```python
from build123d import *

# Parameters (mm, degrees)
SKETCH1_W           = 21.5
SKETCH1_H           = 43
BOSS_EXTRUDE1_DEPTH = 5
CUT_EXTRUDE1_DEPTH  = 5
SKETCH7_W           = 18.5
SKETCH7_H           = 15
BOSS_EXTRUDE2_DEPTH = 5
SKETCH8_R           = 1.175
CUT_EXTRUDE4_DEPTH  = 8
CUT_EXTRUDE5_REACH  = 38.644
SKETCH11_R          = 1.25
CUT_EXTRUDE6_REACH  = 38.644
SKETCH3_R           = 1.5
SKETCH12_R          = 2.25
CUT_EXTRUDE7_DEPTH  = 2
CHAMFER1_SIZE       = 8
CUT_EXTRUDE8_REACH  = 38.644
FILLET4_R           = 2
FILLET5_R           = 5
SKETCH17_W          = 10
SKETCH17_H          = 4
BOSS_EXTRUDE3_DEPTH = 11
FILLET6_R           = 2


with BuildPart() as part:
    # Sketch1 → Boss-Extrude1 (new body)
    with BuildSketch(Plane.XY):
        Rectangle(SKETCH1_W, SKETCH1_H)
    extrude(amount=BOSS_EXTRUDE1_DEPTH)

    # Sketch2 → Cut-Extrude1 (cut)
    with BuildSketch(Plane.XY.offset(5)):
        with BuildLine():
            Line((-6.75, 12.499561173), (-10.75, 12.499561173))
            Line((-10.75, 12.499561173), (-10.75, 21.5))
            Line((-10.75, 21.5), (-3.25, 21.5))
            Line((-3.25, 21.5), (-3.25, 15.944574555))
            ThreePointArc((-3.25, 15.944574555), (-4.294490012, 13.505297076), (-6.75, 12.499561173))
        make_face()
    extrude(amount=-CUT_EXTRUDE1_DEPTH, mode=Mode.SUBTRACT)

    # Sketch7 → Boss-Extrude2 (add)
    with BuildSketch(Plane.XY.offset(5)):
        with Locations((20, 14)):
            Rectangle(SKETCH7_W, SKETCH7_H)
    extrude(amount=-BOSS_EXTRUDE2_DEPTH)

    # Sketch8 → Cut-Extrude4 (cut)
    with BuildSketch(Plane(origin=(29.25, 0, 0), x_dir=(0, 0, -1), z_dir=(1, 0, 0))):
        with Locations((-2.5, 9.5)):
            Circle(SKETCH8_R)
        with Locations((-2.5, 18.5)):
            Circle(SKETCH8_R)
    extrude(amount=-CUT_EXTRUDE4_DEPTH, mode=Mode.SUBTRACT)

    # Sketch11 → Cut-Extrude5 (cut, up to next)
    with BuildSketch(Plane.XY.offset(5), mode=Mode.PRIVATE) as cut_extrude5_sk1:
        with Locations((5, 4.194574555)):
            Circle(SKETCH11_R)
    cut_extrude5_tool1 = extrude(cut_extrude5_sk1.sketch, amount=-CUT_EXTRUDE5_REACH, mode=Mode.PRIVATE) & part.part
    # Sketch11 → Cut-Extrude5 (cut, up to next)
    with BuildSketch(Plane.XY.offset(5), mode=Mode.PRIVATE) as cut_extrude5_sk2:
        with Locations((-7.5, 4.194574555)):
            Circle(SKETCH11_R)
    cut_extrude5_tool2 = extrude(cut_extrude5_sk2.sketch, amount=-CUT_EXTRUDE5_REACH, mode=Mode.PRIVATE) & part.part
    # Sketch11 → Cut-Extrude5 (cut, up to next)
    with BuildSketch(Plane.XY.offset(5), mode=Mode.PRIVATE) as cut_extrude5_sk3:
        with Locations((5, 18.194574555)):
            Circle(SKETCH11_R)
    cut_extrude5_tool3 = extrude(cut_extrude5_sk3.sketch, amount=-CUT_EXTRUDE5_REACH, mode=Mode.PRIVATE) & part.part
    add(cut_extrude5_tool1.solids().sort_by_distance((5, 4.194575, 5))[0], mode=Mode.SUBTRACT)
    add(cut_extrude5_tool2.solids().sort_by_distance((-7.5, 4.194575, 5))[0], mode=Mode.SUBTRACT)
    add(cut_extrude5_tool3.solids().sort_by_distance((5, 18.194575, 5))[0], mode=Mode.SUBTRACT)

    # Sketch3 → Cut-Extrude6 (cut, up to next)
    with BuildSketch(Plane.XY.offset(5), mode=Mode.PRIVATE) as cut_extrude6_sk1:
        with Locations((-7.25, -19)):
            Circle(SKETCH3_R)
    cut_extrude6_tool1 = extrude(cut_extrude6_sk1.sketch, amount=-CUT_EXTRUDE6_REACH, mode=Mode.PRIVATE) & part.part
    # Sketch3 → Cut-Extrude6 (cut, up to next)
    with BuildSketch(Plane.XY.offset(5), mode=Mode.PRIVATE) as cut_extrude6_sk2:
        with Locations((7.25, -19)):
            Circle(SKETCH3_R)
    cut_extrude6_tool2 = extrude(cut_extrude6_sk2.sketch, amount=-CUT_EXTRUDE6_REACH, mode=Mode.PRIVATE) & part.part
    add(cut_extrude6_tool1.solids().sort_by_distance((-7.25, -19, 5))[0], mode=Mode.SUBTRACT)
    add(cut_extrude6_tool2.solids().sort_by_distance((7.25, -19, 5))[0], mode=Mode.SUBTRACT)

    # Sketch12 → Cut-Extrude7 (cut)
    with BuildSketch(Plane(origin=(0, 0, 0), x_dir=(-1, 0, 0), z_dir=(0, 0, -1))):
        with Locations((-5, 4.194574555)):
            Circle(SKETCH12_R)
        with Locations((-5, 18.194574555)):
            Circle(SKETCH12_R)
        with Locations((7.5, 4.194574555)):
            Circle(SKETCH12_R)
    extrude(amount=-CUT_EXTRUDE7_DEPTH, mode=Mode.SUBTRACT)

    # Chamfer1
    chamfer1_edges = [part.edges().sort_by_distance(p)[0] for p in [
        (10.75, 6.5, 2.5),
    ]]
    chamfer(chamfer1_edges, length=CHAMFER1_SIZE)

    # Sketch14 → Cut-Extrude8 (cut, up to next)
    with BuildSketch(Plane.XY.offset(5), mode=Mode.PRIVATE) as cut_extrude8_sk1:
        with BuildLine():
            Line((-10.75, 10.5), (-6.75, 10.5))
            ThreePointArc((-6.75, 10.5), (-2.860912703, 12.110912703), (-1.25, 16))
            Line((-1.25, 16), (-1.25, 21.5))
            Line((-1.25, 21.5), (-10.75, 21.5))
            Line((-10.75, 21.5), (-10.75, 10.5))
        make_face()
    cut_extrude8_tool1 = extrude(cut_extrude8_sk1.sketch, amount=-CUT_EXTRUDE8_REACH, mode=Mode.PRIVATE) & part.part
    add(cut_extrude8_tool1.solids().sort_by_distance((-6.23325, 16.282927, 5))[0], mode=Mode.SUBTRACT)

    # Fillet4
    fillet4_edges = [part.edges().sort_by_distance(p)[0] for p in [
        (-1.25, 21.5, 2.5),
        (-10.75, 10.5, 2.5),
    ]]
    fillet(fillet4_edges, radius=FILLET4_R)

    # Fillet5
    fillet5_edges = [part.edges().sort_by_distance(p)[0] for p in [
        (18.75, 6.5, 2.5),
        (10.75, -1.5, 2.5),
    ]]
    fillet(fillet5_edges, radius=FILLET5_R)

    # Sketch17 → Boss-Extrude3 (add)
    with BuildSketch(Plane.XY.offset(5)):
        with Locations((5.75, 23.5)):
            Rectangle(SKETCH17_W, SKETCH17_H)
    extrude(amount=-BOSS_EXTRUDE3_DEPTH)

    # Fillet6
    fillet6_edges = [part.edges().sort_by_distance(p)[0] for p in [
        (0.75, 21.5, 2.5),
        (10.75, 21.5, 2.5),
        (10.75, 25.5, -0.5),
        (0.75, 25.5, -0.5),
    ]]
    fillet(fillet6_edges, radius=FILLET6_R - 0.0001)  # a hair under: the kernel refuses the full size


solid = part.part
```
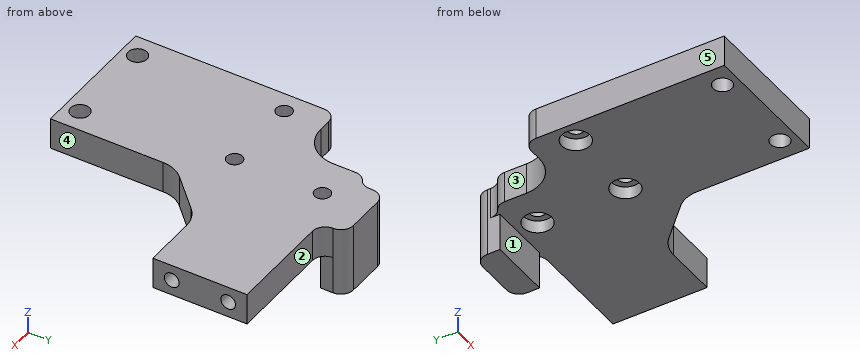
CAD build for the part. Positions are in the model's coordinates, mm. Face numbers are marked on the shaded views. A direction names the side the tool comes from. Round coordinates to 2 decimals unless told otherwise and drop trailing zeros. Order: outer loops, then holes, each group sorted by start corner. A loop starts at its lowest first (then second) coordinate and runs counter-clockwise, first axis right, second up.
Item 1: Probe line 1 along Y through (x, z) = (5, 4.25); line 2 along Y through (x, z) = (5, 1.5); line 3 along X through (y, z) = (3.5, 3.5). List the from-to ranges inside material, lowest first.
Item 2: Saw through at B-B on x = 5. Write the cut outline in (y, z), then the cut area to 3 significant figures.
Item 3: Pin check, flat tips, straight feed: pin 1 (2 mm diameter, centred on x = 5, y = 18.19, fed in from -Z); pin 2 (2.5 mm diameter, centred on x = 20, z = 2, fed in from +Y); pin 3 (0.7 mm diameter, centred on y = 9.5, z = 2.5, fed in from +X); pin 4 (20 mm diameter, centred on x = 7.5, y = 6, fed in from -Z). Stop position of each tip, or through.
Item 4: Saw through at D-D on z = -4.75. Write the cut outline in (x, y), then the cut area to 3 significant figures.
Item 5: Saw through at A-A on y = -19. Write the cut outline in (x, z).
Item 6: Saw through at C-C on x = 22. Write the cut outline in (y, z) (3 decimals), then the cut area to 3 significant figures.
Item 7: Tool access for the marked faces 1, 2, 3, 4 and 5: list every direction of +Z, -Z, +X, -X, +Y, -Y with a clear straight run to the whole face (end or side of a thin tool).
Reported:
1. line 1: y = -21.5 to 2.94, 5.44 to 16.94, 19.44 to 25.5
1. line 2: y = -21.5 to 1.94, 6.44 to 15.94, 20.44 to 25.5
1. line 3: x = -10.75 to -8.54, -6.46 to 3.96, 6.04 to 15.75
2. outline: (-21.5, 0) - (1.94, 0) - (1.94, 2) - (2.94, 2) - (2.94, 5) - (-21.5, 5) - close; (5.44, 2) - (6.44, 2) - (6.44, 0) - (15.94, 0) - (15.94, 2) - (16.94, 2) - (16.94, 5) - (5.44, 5) - close; (19.44, 2) - (20.44, 2) - (20.44, 0) - (21.5, 0) - (21.5, -6) - (25.5, -6) - (25.5, 5) - (19.44, 5) - close
2. area: 226 mm2
3. pin 1: passes through
3. pin 2: stops at y = 21.5
3. pin 3: stops at x = 21.25
3. pin 4: stops at z = 0
4. outline: (0.75, 21.5) - (10.75, 21.5) - (10.75, 23.5) arc R2 ccw to (8.75, 25.5) - (2.75, 25.5) arc R2 ccw to (0.75, 23.5) - close
4. area: 38.3 mm2
5. outline: (-10.75, 0) - (-8.75, 0) - (-8.75, 5) - (-10.75, 5) - close; (-5.75, 0) - (5.75, 0) - (5.75, 5) - (-5.75, 5) - close; (8.75, 0) - (10.75, 0) - (10.75, 5) - (8.75, 5) - close
6. outline: (6.5, 0) - (21.5, 0) - (21.5, 5) - (6.5, 5) - close; hole circle Ø2.35 at (9.5, 2.5); hole circle Ø2.35 at (18.5, 2.5)
6. area: 66.3 mm2
7. face 1: -Z, +X, -X, -Y
7. face 2: +Z, -Z, +X, +Y
7. face 3: +Z, -Z, -X, +Y
7. face 4: +Z, -Z, +X, -Y
7. face 5: +Z, -Z, -X, +Y, -Y
